from build123d import *

# Parameters (mm, degrees)
SKETCH1_R           = 4.25
BOSS_EXTRUDE1_DEPTH = 7
SKETCH2_R           = 4.5
BOSS_EXTRUDE2_DEPTH = 21
SKETCH3_R           = 10.583681917
BOSS_EXTRUDE3_DEPTH = 4
SKETCH8_R           = 1
CUT_EXTRUDE1_DEPTH  = 4


with BuildPart() as part:
    # Sketch1 → Boss-Extrude1 (new body)
    with BuildSketch(Plane.XY):
        with Locations((21, 71.5)):
            Circle(SKETCH1_R)
    extrude(amount=BOSS_EXTRUDE1_DEPTH)

    # Sketch2 → Boss-Extrude2 (add)
    with BuildSketch(Plane.XY.offset(7)):
        with Locations((21, 71.5)):
            Circle(SKETCH2_R)
    extrude(amount=BOSS_EXTRUDE2_DEPTH)

    # Sketch3 → Boss-Extrude3 (add)
    with BuildSketch(Plane.XY.offset(28)):
        with Locations((21, 71.5)):
            Circle(SKETCH3_R)
    extrude(amount=-BOSS_EXTRUDE3_DEPTH)

    # Sketch6 → Cut-Revolve1 (revolve, cut)
    with BuildSketch(Plane(origin=(0, 71.5, 0), x_dir=(1, 0, 0), z_dir=(0, 1, 0))):
        with BuildLine():
            Line((31.583681917, -26.5), (31.583681917, -25.5))
            Line((31.583681917, -25.5), (30.583681917, -25.5))
            ThreePointArc((30.583681917, -25.5), (30.083681917, -26), (30.583681917, -26.5))
            Line((30.583681917, -26.5), (31.583681917, -26.5))
        make_face()
    revolve(axis=Axis((21, 71.5, 28), (0, 0, -1)), mode=Mode.SUBTRACT)

    # Sketch8 → Cut-Extrude1 (cut)
    with BuildSketch(Plane(origin=(0, 0, 24), x_dir=(-1, 0, 0), z_dir=(0, 0, -1))):
        with Locations((-13, 71.5)):
            Circle(SKETCH8_R)
    extrude(amount=-CUT_EXTRUDE1_DEPTH, mode=Mode.SUBTRACT)


solid = part.part
Can you work these out from the model? Positions are in its coordinate system, mm. A direction names the side the tool comes from. Give positions to 0.01 mm unless a question says otherwise; leave off trailing zeros. Loops run counter-clockwise (first coordinate to the right, second up) from the corner with the lowest first, then second, coordinate; pieces in that order, holes last. Notation, with made-up numbers: (-12.75, 9.5) - (3.25, 9.5) arc R31 ccw to (3.25, 36.5) - close; hole circle Ø11 at (-28, 27.5). An arc over 180 degrees is marked (long way). Return JSON: item names as keys, results as strings.
1. For faces 1 (the face through (20.41, 75.96, 15.38)), 2 (the face through (19.622, 81.994, 24.76)), 3 (the face through (18.6, 62, 25.5)), which set-ups out of +Z, -Z, +X, -X, +Y, -Y let a thin tool reach every point of the face, with its end or its side?
Output values:
{"face 1": "-Z", "face 2": "+Z, -Z", "face 3": "none"}
2. I want a section at B-B on x = 21. Please give me the cut outline in (y, z).
Output values:
{"outline": "(60.92, 24) - (67, 24) - (67, 7) - (67.25, 7) - (67.25, 0) - (75.75, 0) - (75.75, 7) - (76, 7) - (76, 24) - (82.08, 24) - (82.08, 25.5) - (81.08, 25.5) arc R0.5 cw to (81.08, 26.5) - (82.08, 26.5) - (82.08, 28) - (60.92, 28) - (60.92, 26.5) - (61.92, 26.5) arc R0.5 cw to (61.92, 25.5) - (60.92, 25.5) - close"}
3. I want a section at C-C on z = 8. Please give me the cut outline in (x, y).
Output values:
{"outline": "circle Ø9 at (21, 71.5)"}
4. I'm going to push flat-ended pins straight in: pin 1 Ø2.5 at (x, y) = (13, 71.5) entering from -Z; pin 2 Ø1.5 at (y, z) = (69, 8) entering from +X; pin 3 Ø6 at (x, z) = (20.5, 13) entering from +Y. Where does each tip first touch, or does it pass through?
Output values:
{"pin 1": "stops at z = 24", "pin 2": "stops at x = 25.15", "pin 3": "stops at y = 76"}
5. If I drill on line 1 (Y direction, x = 13, z = 25.7); line 2 (Z direction, x = 24.5, y = 62); line 3 (X direction, y = 71.5, z = 27.1), over which ranges is the centre line in solid material (lowest first)?
Output values:
{"line 1": "y = 66.99 to 70.5, 72.5 to 76.01", "line 2": "z = 24 to 25.5, 26.5 to 28", "line 3": "x = 10.42 to 12, 14 to 31.58"}
6. We'd pull the mould along Y, two halves only. Please class faces 4 (the face through (19.622, 81.994, 27.26)), 5 (the face through (23.4, 62, 26.5)), 6 (the face through (12.54, 70.61, 25.97)): +Y half, -Y half, draft (parallel to the pull), parting line (faces both ways), or undercut.
Output values:
{"face 4": "parting line", "face 5": "draft", "face 6": "undercut"}
7. I want a section at A-A on y = 71.5. Please give me the cut outline in (x, z), and give its area (3 significant figures).
Output values:
{"outline": "(10.42, 24) - (12, 24) - (12, 28) - (10.42, 28) - (10.42, 26.5) - (11.42, 26.5) arc R0.5 cw to (11.42, 25.5) - (10.42, 25.5) - close; (14, 24) - (16.5, 24) - (16.5, 7) - (16.75, 7) - (16.75, 0) - (25.25, 0) - (25.25, 7) - (25.5, 7) - (25.5, 24) - (31.58, 24) - (31.58, 25.5) - (30.58, 25.5) arc R0.5 cw to (30.58, 26.5) - (31.58, 26.5) - (31.58, 28) - (14, 28) - close", "area": "286 mm²"}
8. I want a section at D-D on z = 4.75. Please give me the cut outline in (x, y), and give its area (3 significant figures).
Output values:
{"outline": "circle Ø8.5 at (21, 71.5)", "area": "56.7 mm²"}
